Autodesk Inventor part; units mm, degrees
ref_plane "YZ Plane" through (0, 0, 0) normal (1, 0, 0) x (0, 1, 0)
ref_plane "XZ Plane" through (0, 0, 0) normal (0, 1, 0) x (-1, 0, 0)
ref_plane "XY Plane" through (0, 0, 0) normal (0, 0, 1) x (1, 0, 0)
sketch "Sketch1" plane through (0, 0, 0) normal (0, 0, 1) x (1, 0, 0)
  line L0 (0, 0) -> (127, 0)
  line L1 (127, 0) -> (127, 40.64)
  line L2 (127, 40.64) -> (0, 40.64)
  line L3 (0, 40.64) -> (0, 0)
  line L4 (0, 40.64) -> (0, 53.34)
  arc A0 (10.16, 63.5) -> (0, 53.34) centre (10.16, 53.34) ccw
  line L5 (10.16, 63.5) -> (40.64, 63.5)
  line L6 (40.64, 63.5) -> (63.5, 40.64)
  point P0 (63.5, 0)
  dimension "width" = 127
  dimension "height" = 63.5
  dimension "d2" = 10.16
  dimension "d3" = 45
  dimension "base_height" = 40.64
extrude "Extrusion1" add sketch "Sketch1" along normal blind 21.59
sketch "Sketch3" plane through (0, 0, 0) normal (-1, 0, 0) x (0, 0, 1)
  line L0 (18.1273, 63.5) -> (3.4627, 63.5)
  line L1 (3.4627, 63.5) -> (10.795, 50.8)
  line L2 (10.795, 50.8) -> (18.1273, 63.5)
  line L3 (0, 0) -> (21.59, 0)
  line L4 (0, 63.5) -> (21.59, 63.5)
  point P0 (10.795, 0)
  dimension "d20" = 12.7
extrude "Extrusion2" cut sketch "Sketch3" against normal through all
sketch "Sketch2" plane through (0, 0, 21.59) normal (0, 0, 1) x (1, 0, 0)
  line L0 (0, 53.34) -> (0, 0)
  line L1 (0, 0) -> (127, 0)
  point P0 (12.7, 20.32)
  dimension "pat_offset" = 12.7
  dimension "d9" = 20.32
hole "Hole1" at (12.7, 20.32, 21.59) direction (0, 0, -1) diameter 5.7912 end through all countersink diameter 11.1252 countersink angle 82
pattern_linear "Rectangular Pattern1" count 4 spacing 25.4 along (1, 0, 0) of "Hole1"
equation "\"height\" = 0.5 * width"
properties part number "Parameter part" material "Steel"
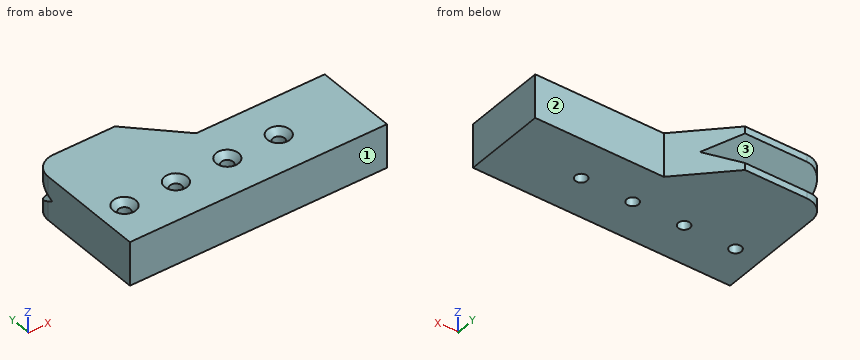
Model file for the job. Use its own axes, mm. Face numbers are marked on the shaded views. A direction names the side the tool comes from. Give positions to 0.01 mm unless a question says otherwise; leave off trailing zeros. Order: outer loops, then holes, each group sorted by start corner. A loop starts at its lowest first (then second) coordinate and runs counter-clockwise, first axis right, second up. Notation, with made-up numbers: (-12.5, 59) - (30.5, 59) arc R17 ccw to (30.5, 68) - close; hole circle Ø10 at (3, -13.75). An arc over 180 degrees is marked (long way). Write item = value, one per line. Start each with the question number.
1. Drop flat-ended pins along their axis: P1, Ø11, axis at x = 81, z = 7, coming from the +Y side; P2, Ø6.5, axis at x = 88.9, y = 20.32, coming from the +Z side; P3, Ø5, axis at x = 55.5, z = 9.5, coming from the +Y side. Give the stop position or say it passes through.
2. Cut at C-C, the plane y = 57.5. List the corners of the cut face in (x, z).
3. Which spindle directions (+Z, -Z, +X, -X, +Y, -Y) get a long thin tool onto all of the face, cutting with end or side? Do the marked faces 1, 2 and 3. Say none if no direction does.
4. Cut at A-A, the plane y = 20.32. List the corners of the cut face in (x, z), and give its area (3 significant figures).
5. Cut at B-B, the plane x = 12.7. List the corners of the cut face in (y, z) (3 decimals).
6. Cut at D-D, the plane z = 16.5. List the corners of the cut face in (x, y), and give its area (3 significant figures).
7. Probe line 1 along Y through (x, z) = (88.9, 12.5); line 2 along X through (y, z) = (20.32, 10); line 3 along Y through (x, z) = (83, 14.5). List the from-to ranges inside material, lowest first.
Taken from the geometry:
q1.P1 = 40.64
q1.P2 = 18.93
q1.P3 = 51.14
q2.outline = (0.89, 0) - (46.64, 0) - (46.64, 6.93) - (0.89, 6.93) - close; (0.89, 14.66) - (46.64, 14.66) - (46.64, 21.59) - (0.89, 21.59) - close
q3.face_1 = +Z, -Z, +X, -X, -Y
q3.face_2 = +Z, -Z, +X, +Y
q3.face_3 = +X, -X, +Y
q4.outline = (0, 0) - (9.8, 0) - (9.8, 18.52) - (7.14, 21.59) - (0, 21.59) - close; (15.6, 0) - (35.2, 0) - (35.2, 18.52) - (32.54, 21.59) - (18.26, 21.59) - (15.6, 18.52) - close; (41, 0) - (60.6, 0) - (60.6, 18.52) - (57.94, 21.59) - (43.66, 21.59) - (41, 18.52) - close; (66.4, 0) - (86, 0) - (86, 18.52) - (83.34, 21.59) - (69.06, 21.59) - (66.4, 18.52) - close; (91.8, 0) - (127, 0) - (127, 21.59) - (94.46, 21.59) - (91.8, 18.52) - close
q4.area = 2,210 mm²
q5.outline = (0, 0) - (17.424, 0) - (17.424, 18.522) - (14.757, 21.59) - (0, 21.59) - close; (23.216, 0) - (63.5, 0) - (63.5, 3.463) - (50.8, 10.795) - (63.5, 18.127) - (63.5, 21.59) - (25.883, 21.59) - (23.216, 18.522) - close
q6.outline = (0, 0) - (127, 0) - (127, 40.64) - (63.5, 40.64) - (43.46, 60.68) - (3.14, 60.68) arc R10.16 ccw to (0, 53.34) - close; hole circle Ø5.79 at (12.7, 20.32); hole circle Ø5.79 at (38.1, 20.32); hole circle Ø5.79 at (63.5, 20.32); hole circle Ø5.79 at (88.9, 20.32)
q6.area = 6,120 mm²
q7.line_1 = 0 to 17.42, 23.22 to 40.64
q7.line_2 = 0 to 9.8, 15.6 to 35.2, 41 to 60.6, 66.4 to 86, 91.8 to 127
q7.line_3 = 0 to 40.64
